from build123d import *

# Parameters (mm, degrees)
F0_R     = 1.5
F1_DEPTH = 2.5
F2_DEPTH = 5
F3_R     = 0.99999
F6_DEPTH = 1.1
F7_D     = 2.2
F7_DEPTH = 2.501
F8_D     = 2.2


# Not quite as in the source:
# - a fillet or chamfer is up to 0.001 mm smaller than in the source, because OpenCascade refuses the exact size


with BuildPart() as f1:
    # F0 (on Front) → F1 (new body, symmetric)
    with BuildSketch(Plane.XZ):
        with BuildLine():
            ThreePointArc((-7.4377474476, -3.8639245472), (-7.4497190923, -7.3994381845), (-3.9142054549, -7.4114098292))
            Line((-3.9142054549, -7.4114098292), (18.78970035, 15.1392589236))
            ThreePointArc((18.78970035, 15.1392589236), (18.8016719947, 18.6747725609), (15.2661583574, 18.6867442056))
            Line((15.2661583574, 18.6867442056), (-7.4377474476, -3.8639245472))
        make_face()
        Circle(F0_R, mode=Mode.SUBTRACT)
        Circle(F0_R)
    extrude(amount=F1_DEPTH, both=True)

    # F0 (on Front) → F2 (cut, symmetric)
    with BuildSketch(Plane.XZ):
        Circle(F0_R)
    extrude(amount=F2_DEPTH, both=True, mode=Mode.SUBTRACT)

    # F3 (radius 1 in the source; OpenCascade refuses exactly that, so slightly less here)
    f3_edges = [f1.edges().sort_by_distance(p)[0] for p in [
        (3.914205, -2.5, 7.41141),
        (3.914205, 2.5, 7.41141),
    ]]
    fillet(f3_edges, radius=F3_R)

    # F5 (on Front) → F6 (cut, symmetric)
    with BuildSketch(Plane.XZ):
        Polygon((17.2437955285, 15.4185445413), (16.6082652356, 13.0784374397), (14.2639078916, 12.4587692675), (15.1712653624, 11.5452460911), (18.1511529993, 14.5050213649), align=None)
        Polygon((14.2639078916, 12.4587692675), (16.6082652356, 13.0784374397), (17.2437955285, 15.4185445413), (15.5349684774, 17.1389834706), (13.1906111334, 16.5193152984), (12.5550808405, 14.1792081968), align=None)
        Polygon((11.6477233698, 15.0927313731), (12.5550808405, 14.1792081968), (13.1906111334, 16.5193152984), (15.5349684774, 17.1389834706), (14.6276110067, 18.0525066469), align=None)
    extrude(amount=F6_DEPTH, both=True, mode=Mode.SUBTRACT)

    # F7 (through all, one way)
    with BuildSketch(Plane.XZ):
        with Locations((14.8994381845, 14.798876369)):
            Circle(F7_D / 2)
    extrude(amount=-F7_DEPTH, mode=Mode.SUBTRACT)

    # F8 (through all)
    with Locations(Plane(origin=(0, 0, 0), x_dir=(1, 0, 0), z_dir=(0, 1, 0))):
        with Locations((14.8994381845, -14.798876369)):
            Hole(F8_D / 2)


solid = f1.part
Could you check a few things on this model? Use its own coordinates, in mm. A direction names the side the tool comes from. Give positions to 0.01 mm unless a question says otherwise; leave off trailing zeros. Order: outer loops, then holes, each group sorted by start corner. A loop starts at its lowest first (then second) coordinate and runs counter-clockwise, first axis right, second up.
1. Suppose I cut it at A-A (y = -0.3). List the corners of the cut face in (x, z) for me, plus the area to 3 significant figures.
2. We'd pull the mould along X, two halves only. Please class faces 3 (the flat face through (7.28, -0.02, 3.71)), 4 (the flat face through (16.3, -1.1, 14.8)), 5 (the flat face through (6, 2.5, 6)): pulls with the +X half, pulls with the -X half, needs draft (parallel to the pull), parting line crosses it, or undercut.
3. I need wall thicknesses on L1, parallel to Z at x = -0.5, y = -1.9; L2, parallel to X at y = 0.85, z = 0.5; L3, parallel to Z at x = -1.25, y = -0.4. Which ranges of each line are inside material? Lowest first, please.
4. For faces 1 (the flat face through (16.3, 1.1, 14.8)), 2 (the cylindrical face through (7.385, 2.215, 4.235)), which set-ups out of +Z, -Z, +X, -X, +Y, -Y let a thin tool reach every point of the face, with its end or its side?
5. Will these pins go through, and if not, where does the flat tip stop? P1, Ø1, axis at y = 1.5, z = -3, coming from the +X side; P2, Ø2, axis at x = 14.9, z = 14.8, coming from the +Y side; P3, Ø1, axis at x = 6.5, y = 1.5, coming from the +Z side.
Solved:
1. outline: (-7.44, -3.86) arc R2.5 ccw to (-3.91, -7.41) - (15.17, 11.55) - (11.65, 15.09) - close; (14.63, 18.05) - (18.15, 14.51) - (18.79, 15.14) arc R2.5 ccw to (15.27, 18.69) - close; hole circle Ø3 at (0, 0)
1. area: 152 mm2
2. face 3: pulls with the +X half
2. face 4: undercut
2. face 5: needs draft
3. L1: z = -3.9 to -1.41, 1.41 to 2.91
3. L2: x = -3.04 to -1.41, 1.41 to 4.05
3. L3: z = -4.77 to -0.83, 0.83 to 2.28
4. face 1: none
4. face 2: -Z, +X, +Y
5. P1: stops at x = 1.03
5. P2: passes through
5. P3: stops at z = 10.48
